from build123d import *

# Parameters (mm, degrees)
SKETCH2_W               = 84
SKETCH2_H               = 48.2
BOSS_EXTRUDE1_DEPTH     = 3
SKETCH3_W               = 3.8
SKETCH3_H               = 48.2
BOSS_EXTRUDE2_DEPTH     = 19
SKETCH4_W               = 4
SKETCH4_H               = 48.2
BOSS_EXTRUDE3_DEPTH     = 13
BOSS_EXTRUDE4_DEPTH     = 7.5
SKETCH6_W               = 3
SKETCH6_H               = 48.2
CUT_EXTRUDE1_DEPTH      = 9
SKETCH7_W               = 68
SKETCH7_H               = 40.2
CUT_EXTRUDE2_DEPTH      = 0.5
SKETCH9_W               = 84
SKETCH9_H               = 48.2
BOSS_EXTRUDE5_DEPTH     = 15.4
CUT_EXTRUDE3_DEPTH      = 53.202107237
CUT_EXTRUDE3_DEPTH_BACK = 14
CUT_EXTRUDE4_DEPTH      = 53.202107237
CUT_EXTRUDE4_DEPTH_BACK = 53.202107237
FILLET1_R               = 3
SKETCH12_W              = 76.4
SKETCH12_H              = 4.2
CUT_EXTRUDE5_DEPTH      = 20
CUT_EXTRUDE6_DEPTH      = 53.202107283
CUT_EXTRUDE6_DEPTH_BACK = 2
SKETCH13_W              = 68.4
SKETCH13_H              = 41.8


with BuildPart() as part:
    # Sketch2 → Boss-Extrude1 (new body)
    with BuildSketch(Plane(origin=(0, 0, 0), x_dir=(1, 0, 0), z_dir=(0, 1, 0))):
        Rectangle(SKETCH2_W, SKETCH2_H)
    extrude(amount=BOSS_EXTRUDE1_DEPTH)

    # Sketch3 → Boss-Extrude2 (add)
    with BuildSketch(Plane(origin=(0, 3, 0), x_dir=(1, 0, 0), z_dir=(0, 1, 0))):
        with Locations((-40.1, 0)):
            Rectangle(SKETCH3_W, SKETCH3_H)
        with Locations((40.1, 0)):
            Rectangle(SKETCH3_W, SKETCH3_H)
    extrude(amount=BOSS_EXTRUDE2_DEPTH)

    # Sketch4 → Boss-Extrude3 (add)
    with BuildSketch(Plane(origin=(0, 3, 0), x_dir=(1, 0, 0), z_dir=(0, 1, 0))):
        with Locations((-36.2, 0)):
            Rectangle(SKETCH4_W, SKETCH4_H)
        with Locations((36.2, 0)):
            Rectangle(SKETCH4_W, SKETCH4_H)
    extrude(amount=BOSS_EXTRUDE3_DEPTH)

    # Sketch5 → Boss-Extrude4 (add, symmetric)
    with BuildSketch(Plane(origin=(0, 0, 0), x_dir=(-1, 0, 0), z_dir=(0, 0, -1))):
        Polygon((-38.2, 20), (-37.4, 18), (-38.2, 18), align=None)
    boss_extrude4 = extrude(amount=BOSS_EXTRUDE4_DEPTH, both=True)

    # Sketch6 → Cut-Extrude1 (cut)
    with BuildSketch(Plane(origin=(0, 16, 0), x_dir=(1, 0, 0), z_dir=(0, 1, 0))):
        with Locations((35.7, 0)):
            Rectangle(SKETCH6_W, SKETCH6_H)
        with Locations((-35.7, 0)):
            Rectangle(SKETCH6_W, SKETCH6_H)
    extrude(amount=-CUT_EXTRUDE1_DEPTH, mode=Mode.SUBTRACT)

    # Mirror1: Boss-Extrude4 across plane
    add(boss_extrude4.mirror(Plane(origin=(0, 0, 0), x_dir=(0, 0, 1), z_dir=(1, 0, 0))))

    # Sketch7 → Cut-Extrude2 (cut)
    with BuildSketch(Plane(origin=(0, 3, 0), x_dir=(1, 0, 0), z_dir=(0, 1, 0))):
        Rectangle(SKETCH7_W, SKETCH7_H)
    extrude(amount=-CUT_EXTRUDE2_DEPTH, mode=Mode.SUBTRACT)

    # Sketch9 → Boss-Extrude5 (add)
    with BuildSketch(Plane(origin=(0, 2.5, 0), x_dir=(1, 0, 0), z_dir=(0, 1, 0))):
        Rectangle(SKETCH9_W, SKETCH9_H)
    extrude(amount=-BOSS_EXTRUDE5_DEPTH)

    # Sketch10 → Cut-Extrude3 (cut, two sides: drawn at the far end of the back side and taken through both)
    with BuildSketch(Plane(origin=(0, 2.5, 0), x_dir=(1, 0, 0), z_dir=(0, 1, 0)).offset(-CUT_EXTRUDE3_DEPTH_BACK)):
        with BuildLine():
            Line((25.1, 3.7), (25.1, 12.1))
            ThreePointArc((25.1, 12.1), (29.6, 16.6), (34.1, 12.1))
            Line((34.1, 12.1), (34.1, 3.7))
            ThreePointArc((34.1, 3.7), (29.6, -0.8), (25.1, 3.7))
        make_face()
    extrude(amount=CUT_EXTRUDE3_DEPTH + CUT_EXTRUDE3_DEPTH_BACK, mode=Mode.SUBTRACT)

    # Sketch11 → Cut-Extrude4 (cut, two sides: drawn at the far end of the back side and taken through both)
    with BuildSketch(Plane(origin=(0, 2.5, 0), x_dir=(1, 0, 0), z_dir=(0, 1, 0)).offset(-CUT_EXTRUDE4_DEPTH_BACK)):
        with BuildLine():
            Line((9.6, 2.2), (9.6, -15.3))
            ThreePointArc((9.6, -15.3), (4.6, -20.3), (-0.4, -15.3))
            Line((-0.4, -15.3), (-0.4, 2.2))
            ThreePointArc((-0.4, 2.2), (4.6, 7.2), (9.6, 2.2))
        make_face()
    extrude(amount=CUT_EXTRUDE4_DEPTH + CUT_EXTRUDE4_DEPTH_BACK, mode=Mode.SUBTRACT)

    # Fillet1
    # the kernel refuses this fillet: 3 mm, written as the material it takes off along each edge
    with BuildSketch(Plane(origin=(-39, -9.9, 21.1), x_dir=(-1, 0, 0), z_dir=(0, -1, 0))) as fillet1_piece_1_section:
        Polygon((0, 0), (FILLET1_R * 1.02, 0), (FILLET1_R * 1.02, -FILLET1_R * 1.02), (0, -FILLET1_R * 1.02), align=None)
    fillet1_piece_1 = extrude(amount=FILLET1_R * 1.02, mode=Mode.PRIVATE)
    fillet1_piece_1 = fillet1_piece_1 - Plane(origin=(-39, -9.9, 21.1), x_dir=(0.7071067811865475, 0, -0.7071067811865476), z_dir=(0, -1, 0)) * Sphere(FILLET1_R, mode=Mode.PRIVATE)
    add(fillet1_piece_1, mode=Mode.SUBTRACT)
    with BuildSketch(Plane(origin=(-39, -9.9, -21.1), x_dir=(0, -1, 0), z_dir=(0, 0, -1))) as fillet1_piece_2_section:
        Polygon((0, 0), (FILLET1_R * 1.02, 0), (FILLET1_R * 1.02, FILLET1_R * 1.02), (0, FILLET1_R * 1.02), align=None)
    fillet1_piece_2 = extrude(amount=FILLET1_R * 1.02, mode=Mode.PRIVATE)
    fillet1_piece_2 = fillet1_piece_2 - Plane(origin=(-39, -9.9, -21.1), x_dir=(0.7071067811865475, 0.7071067811865475, 0), z_dir=(0, 0, -1)) * Sphere(FILLET1_R, mode=Mode.PRIVATE)
    add(fillet1_piece_2, mode=Mode.SUBTRACT)
    with BuildSketch(Plane(origin=(39, -9.9, -21.1), x_dir=(0, -1, 0), z_dir=(0, 0, -1))) as fillet1_piece_3_section:
        Polygon((0, 0), (FILLET1_R * 1.02, 0), (FILLET1_R * 1.02, -FILLET1_R * 1.02), (0, -FILLET1_R * 1.02), align=None)
    fillet1_piece_3 = extrude(amount=FILLET1_R * 1.02, mode=Mode.PRIVATE)
    fillet1_piece_3 = fillet1_piece_3 - Plane(origin=(39, -9.9, -21.1), x_dir=(-0.7071067811865475, 0.7071067811865475, 0), z_dir=(0, 0, -1)) * Sphere(FILLET1_R, mode=Mode.PRIVATE)
    add(fillet1_piece_3, mode=Mode.SUBTRACT)
    with BuildSketch(Plane(origin=(39, -9.9, 21.1), x_dir=(0, -1, 0), z_dir=(1, 0, 0))) as fillet1_piece_4_section:
        Polygon((0, 0), (FILLET1_R * 1.02, 0), (FILLET1_R * 1.02, -FILLET1_R * 1.02), (0, -FILLET1_R * 1.02), align=None)
    fillet1_piece_4 = extrude(amount=FILLET1_R * 1.02, mode=Mode.PRIVATE)
    fillet1_piece_4 = fillet1_piece_4 - Plane(origin=(39, -9.9, 21.1), x_dir=(0, 0.7071067811865475, -0.7071067811865475), z_dir=(1, 0, 0)) * Sphere(FILLET1_R, mode=Mode.PRIVATE)
    add(fillet1_piece_4, mode=Mode.SUBTRACT)
    with BuildSketch(Plane(origin=(-42, -12.9, 21.1), x_dir=(1, 0, 0), z_dir=(0, 0, -1)), Plane(origin=(42, -12.9, -21.1), x_dir=(-1, 0, 0), z_dir=(0, 0, 1))) as fillet1_piece_5:
        with BuildLine():
            CenterArc((FILLET1_R, -FILLET1_R), FILLET1_R, 90, 90)
            Line((0, -FILLET1_R), (0, 0))
            Line((0, 0), (FILLET1_R, 0))
        make_face()
    extrude(amount=42.2, mode=Mode.SUBTRACT)
    with BuildSketch(Plane(origin=(-39, -12.9, -24.1), x_dir=(0, 1, 0), z_dir=(1, 0, 0))) as fillet1_piece_6:
        with BuildLine():
            CenterArc((FILLET1_R, FILLET1_R), FILLET1_R, 180, 90)
            Line((0, FILLET1_R), (0, 0))
            Line((0, 0), (FILLET1_R, 0))
        make_face()
    extrude(amount=78, mode=Mode.SUBTRACT)
    with BuildSketch(Plane(origin=(39, -12.9, 24.1), x_dir=(0, 0, -1), z_dir=(-1, 0, 0))) as fillet1_piece_7:
        with BuildLine():
            CenterArc((FILLET1_R, -FILLET1_R), FILLET1_R, 90, 90)
            Line((0, -FILLET1_R), (0, 0))
            Line((0, 0), (FILLET1_R, 0))
        make_face()
    extrude(amount=78, mode=Mode.SUBTRACT)
    with BuildSketch(Plane(origin=(25.1, 2.5, -3.7), x_dir=(-1, 0, 0), z_dir=(0, 0, -1))) as fillet1_piece_8:
        with BuildLine():
            CenterArc((FILLET1_R, -FILLET1_R), FILLET1_R, 90, 90)
            Line((0, -FILLET1_R), (0, 0))
            Line((0, 0), (FILLET1_R, 0))
        make_face()
    extrude(amount=8.4, mode=Mode.SUBTRACT)
    with BuildSketch(Plane(origin=(29.6, 2.5, -12.1), x_dir=(-1, 0, 0), z_dir=(0, 0, 1))) as fillet1_piece_9_section:
        with BuildLine():
            CenterArc((4.5 + FILLET1_R, FILLET1_R), FILLET1_R, 180, 90)
            Line((4.5 + FILLET1_R, 0), (4.5, 0))
            Line((4.5, 0), (4.5, FILLET1_R))
        make_face()
    fillet1_piece_9 = revolve(axis=Axis((29.6, 2.5, -12.1), (0, -1, 0)), revolution_arc=263.525069882, mode=Mode.PRIVATE)
    fillet1_piece_9 = split(fillet1_piece_9, bisect_by=Plane(origin=(34, 1.640934382, -17.429209867), z_dir=(-1, 0, 0)), keep=Keep.TOP, mode=Mode.PRIVATE)
    add(fillet1_piece_9, mode=Mode.SUBTRACT)
    with BuildSketch(Plane(origin=(29.6, 2.5, -3.7), x_dir=(0.11276846361504911, 0, -0.9936212928545268), z_dir=(-0.9936212928545268, 0, -0.11276846361504911))) as fillet1_piece_10_section:
        with BuildLine():
            CenterArc((4.5 + FILLET1_R, FILLET1_R), FILLET1_R, 180, 90)
            Line((4.5 + FILLET1_R, 0), (4.5, 0))
            Line((4.5, 0), (4.5, FILLET1_R))
        make_face()
    fillet1_piece_10 = revolve(axis=Axis((29.6, 2.5, -3.7), (0, -1, 0)), revolution_arc=263.525069882, mode=Mode.PRIVATE)
    fillet1_piece_10 = split(fillet1_piece_10, bisect_by=Plane(origin=(34, 1.640934386, 1.629209863), z_dir=(-1, 0, 0)), keep=Keep.TOP, mode=Mode.PRIVATE)
    add(fillet1_piece_10, mode=Mode.SUBTRACT)
    with BuildSketch(Plane(origin=(4.6, 2.5, -2.2), x_dir=(-1, 0, 0), z_dir=(0, 0, 1))) as fillet1_piece_11:
        with BuildLine():
            CenterArc((5 + FILLET1_R, FILLET1_R), FILLET1_R, 180, 90)
            Line((5 + FILLET1_R, 0), (5, 0))
            Line((5, 0), (5, FILLET1_R))
        make_face()
    revolve(axis=Axis((4.6, 2.5, -2.2), (0, -1, 0)), revolution_arc=180, mode=Mode.SUBTRACT)
    with BuildSketch(Plane(origin=(9.6, 2.5, -2.2), x_dir=(0, -1, 0), z_dir=(0, 0, 1)), Plane(origin=(-0.4, 2.5, 15.3), x_dir=(0, -1, 0), z_dir=(0, 0, -1)), Plane(origin=(9.6, -12.9, -2.2), x_dir=(1, 0, 0), z_dir=(0, 0, 1)), Plane(origin=(-0.4, -12.9, 15.3), x_dir=(-1, 0, 0), z_dir=(0, 0, -1))) as fillet1_piece_12:
        with BuildLine():
            CenterArc((FILLET1_R, FILLET1_R), FILLET1_R, 180, 90)
            Line((0, FILLET1_R), (0, 0))
            Line((0, 0), (FILLET1_R, 0))
        make_face()
    extrude(amount=17.5, mode=Mode.SUBTRACT)
    with BuildSketch(Plane(origin=(4.6, 2.5, 15.3), x_dir=(1, 0, 0), z_dir=(0, 0, -1))) as fillet1_piece_13_section:
        with BuildLine():
            CenterArc((5 + FILLET1_R, FILLET1_R), FILLET1_R, 180, 90)
            Line((5 + FILLET1_R, 0), (5, 0))
            Line((5, 0), (5, FILLET1_R))
        make_face()
    fillet1_piece_13 = revolve(axis=Axis((4.6, 2.5, 15.3), (0, -1, 0)), revolution_arc=159.706638681, mode=Mode.PRIVATE)
    fillet1_piece_13 = split(fillet1_piece_13, bisect_by=Plane(origin=(8.507236212, 1.653326519, 20.1), z_dir=(0, 0, -1)), keep=Keep.TOP, mode=Mode.PRIVATE)
    add(fillet1_piece_13, mode=Mode.SUBTRACT)
    with BuildSketch(Plane(origin=(4.6, 2.5, 15.3), x_dir=(0.9379291266520984, 0, 0.3468269790221515), z_dir=(0.3468269790221515, 0, -0.9379291266520984))) as fillet1_piece_14_section:
        with BuildLine():
            CenterArc((5 + FILLET1_R, FILLET1_R), FILLET1_R, 180, 90)
            Line((5 + FILLET1_R, 0), (5, 0))
            Line((5, 0), (5, FILLET1_R))
        make_face()
    fillet1_piece_14 = revolve(axis=Axis((4.6, 2.5, 15.3), (0, -1, 0)), revolution_arc=159.706638681, mode=Mode.PRIVATE)
    fillet1_piece_14 = split(fillet1_piece_14, bisect_by=Plane(origin=(8.773531285, 1.782701888, 20.1), z_dir=(0, 0, -1)), keep=Keep.TOP, mode=Mode.PRIVATE)
    add(fillet1_piece_14, mode=Mode.SUBTRACT)
    with BuildSketch(Plane(origin=(4.6, -12.9, -2.2), x_dir=(-1, 0, 0), z_dir=(0, 0, 1))) as fillet1_piece_15:
        with BuildLine():
            CenterArc((5 + FILLET1_R, -FILLET1_R), FILLET1_R, 90, 90)
            Line((5, -FILLET1_R), (5, 0))
            Line((5, 0), (5 + FILLET1_R, 0))
        make_face()
    revolve(axis=Axis((4.6, -12.9, -2.2), (0, -1, 0)), revolution_arc=180, mode=Mode.SUBTRACT)
    with BuildSketch(Plane(origin=(4.6, -12.9, 15.3), x_dir=(1, 0, 0), z_dir=(0, 0, -1))) as fillet1_piece_16:
        with BuildLine():
            CenterArc((5 + FILLET1_R, -FILLET1_R), FILLET1_R, 90, 90)
            Line((5, -FILLET1_R), (5, 0))
            Line((5, 0), (5 + FILLET1_R, 0))
        make_face()
    revolve(axis=Axis((4.6, -12.9, 15.3), (0, -1, 0)), revolution_arc=180, mode=Mode.SUBTRACT)
    with BuildSketch(Plane(origin=(-42, -9.9, -24.1), x_dir=(1, 0, 0), z_dir=(0, 1, 0)), Plane(origin=(42, 29.5, -24.1), x_dir=(-1, 0, 0), z_dir=(0, -1, 0)), Plane(origin=(42, 29.5, 24.1), x_dir=(0, 0, -1), z_dir=(0, -1, 0)), Plane(origin=(-42, -9.9, 24.1), x_dir=(0, 0, -1), z_dir=(0, 1, 0))) as fillet1_piece_17:
        with BuildLine():
            CenterArc((FILLET1_R, -FILLET1_R), FILLET1_R, 90, 90)
            Line((0, -FILLET1_R), (0, 0))
            Line((0, 0), (FILLET1_R, 0))
        make_face()
    extrude(amount=39.4, mode=Mode.SUBTRACT)

    # Sketch12 → Cut-Extrude5 (cut)
    with BuildSketch(Plane(origin=(0, 2.5, 0), x_dir=(1, 0, 0), z_dir=(0, 1, 0))):
        with Locations((0, 22)):
            Rectangle(SKETCH12_W, SKETCH12_H)
        with Locations((0, -22)):
            Rectangle(SKETCH12_W, SKETCH12_H)
    extrude(amount=CUT_EXTRUDE5_DEPTH, mode=Mode.SUBTRACT)

    # Sketch13 → Cut-Extrude6 (cut, two sides: drawn at the far end of the back side and taken through both)
    with BuildSketch(Plane(origin=(0, 2.5, 0), x_dir=(1, 0, 0), z_dir=(0, 1, 0)).offset(-CUT_EXTRUDE6_DEPTH_BACK)):
        Rectangle(SKETCH13_W, SKETCH13_H)
    extrude(amount=CUT_EXTRUDE6_DEPTH + CUT_EXTRUDE6_DEPTH_BACK, mode=Mode.SUBTRACT)


solid = part.part
Geometry: final body of the model. Coordinates: model frame, mm. A direction names the side the tool comes from. Give positions to 0.01 mm unless a question says otherwise; leave off trailing zeros. Write each loop counter-clockwise with the first axis right and the second up, starting at its lowest first coordinate (ties: lowest second). Pieces come first, ordered by that corner, then holes. Notation, with made-up numbers: (7.5, 53) -> (18.5, 53) arc R22 ccw to (18.5, 60) -> close; hole circle Ø4 at (55, 63.5). An arc over 180 degrees is marked (long way). Answer in a Markdown table with one row per item.
(1) Section query B-B on y = 9. Return loops of the section in (x, z).
Answers below:
| item | result |
|---|---|
| outline | (-42, -21.1) arc R3 ccw to (-39, -24.1) -> (-38.2, -24.1) -> (-38.2, -19.9) -> (-37.2, -19.9) -> (-37.2, 19.9) -> (-38.2, 19.9) -> (-38.2, 24.1) -> (-39, 24.1) arc R3 ccw to (-42, 21.1) -> close; (37.2, -19.9) -> (38.2, -19.9) -> (38.2, -24.1) -> (39, -24.1) arc R3 ccw to (42, -21.1) -> (42, 21.1) arc R3 ccw to (39, 24.1) -> (38.2, 24.1) -> (38.2, 19.9) -> (37.2, 19.9) -> close |
(2) Section query D-D on x = 29.6. Return loops of the section in (y, z), then the cut area to 3 significant figures.
Answers below:
| item | result |
|---|---|
| outline | (-12.9, -21.1) arc R3 ccw to (-9.9, -24.1) -> (2.5, -24.1) -> (2.5, -20.9) -> (0.5, -20.9) -> (0.5, -16.77) arc R3 ccw to (-0.5, -16.6) -> (-11.5, -16.6) -> (-11.5, 0.8) -> (-0.5, 0.8) arc R3 ccw to (0.5, 0.97) -> (0.5, 20.9) -> (2.5, 20.9) -> (2.5, 24.1) -> (-9.9, 24.1) arc R3 ccw to (-12.9, 21.1) -> close |
| area | 446 mm^2 |
(3) Ray query, line 1 along X through (y, z) = (3, 15); line 2 along X through (y, z) = (-3, -4.5); line 3 along X through (y, z) = (10.5, 0.5). Return the intervals inside material, ascending. Write a range as [from, to].
Answers below:
| item | result |
|---|---|
| line 1 | [-42, -34.2], [34.2, 42] |
| line 2 | [-42, 0.16], [9.04, 25.1], [34.1, 42] |
| line 3 | [-42, -37.2], [37.2, 42] |
(4) Draft query along X for faces 4 (the flat face through (37, 6, -19.9)), 5 (the flat face through (-37.8, 19, -0.1)), 6 (the flat face through (42, 6, 0)), 7 (the flat face through (0, -2, -24.1)). Return one class per face: +X half, -X half, draft (parallel to the pull), parting line (faces both ways), or undercut.
Answers below:
| item | result |
|---|---|
| face 4 | undercut |
| face 5 | undercut |
| face 6 | +X half |
| face 7 | draft |
(5) Section query C-C on x = -8. Return loops of the section in (y, z).
Answers below:
| item | result |
|---|---|
| outline | (-12.9, -21.1) arc R3 ccw to (-9.9, -24.1) -> (2.5, -24.1) -> (2.5, -20.9) -> (0.5, -20.9) -> (0.5, 20.9) -> (2.5, 20.9) -> (2.5, 24.1) -> (-9.9, 24.1) arc R3 ccw to (-12.9, 21.1) -> close |
(6) Set-up query: faces 1 (the cylindrical face through (4.7, -4.8, 20.3)), 2 (the flat face through (36, 7, 0)), 3 (the cylindrical face through (29.5, -5.6, -16.6)). Return all of +Z, -Z, +X, -X, +Y, -Y with unobstructed straight access to the full face (end or side cutting, diameter ignored); none if empty.
Answers below:
| item | result |
|---|---|
| face 1 | +Y, -Y |
| face 2 | +Z, -Z, +Y |
| face 3 | +Y |
(7) Pin query (flat end, axial travel): pin 1 (8 mm diameter, centred on x = 33.5, y = 7, fed in from -Z); pin 2 (1.3 mm diameter, centred on x = -15, z = -22, fed in from +Y); pin 3 (1.2 mm diameter, centred on x = 36.5, y = 7.5, fed in from +Z); pin 4 (0.6 mm diameter, centred on x = 38, y = 19, fed in from +Z). Return the tip coordinate at first contact, or that it passes through.
Answers below:
| item | result |
|---|---|
| pin 1 | z = -19.9 |
| pin 2 | y = 2.5 |
| pin 3 | z = 19.9 |
| pin 4 | z = 24.1 |
